The listing builds one solid part. Answer for the finished solid, in the listing's coordinates (mm). Face numbers are marked on the shaded views. A direction names the side the tool comes from. Coordinates: 2 decimals unless noted, no trailing zeros. Write each loop counter-clockwise with the first axis right and the second up, starting at its lowest first coordinate (ties: lowest second). Pieces come first, ordered by that corner, then holes.
from build123d import *

# Parameters (mm, degrees)
BASE_FLANGE1_DEPTH                                  = 50
M12_CLEARANCE_HOLE1_D                               = 12.1
M6_CLEARANCE_HOLE1_D                                = 6.6
BREAK_CORNER1_START                                 = -3
BREAK_CORNER1_DEPTH                                 = 3
BREAK_CORNER1_2_DEPTH                               = 3
EDGE_FLANGE2_DEPTH                                  = 47
CSK_FOR_M8_COUNTERSUNK_FLAT_HEAD_SCREW1_D           = 9
CSK_FOR_M8_COUNTERSUNK_FLAT_HEAD_SCREW1_CSINK_D     = 17.3
CSK_FOR_M8_COUNTERSUNK_FLAT_HEAD_SCREW1_CSINK_ANGLE = 90
CSK_FOR_M6_COUNTERSUNK_FLAT_HEAD_SCREW1_D           = 6.6
CSK_FOR_M6_COUNTERSUNK_FLAT_HEAD_SCREW1_CSINK_D     = 12.6
CSK_FOR_M6_COUNTERSUNK_FLAT_HEAD_SCREW1_CSINK_ANGLE = 90


# Read off the part's stored shape, not the designer's step: Break-Corner1
# Sheet-metal steps are written as plain solids
with BuildPart() as part:
    # Sketch1 → Base-Flange1 (new body)
    with BuildSketch(Plane.XY):
        with BuildLine():
            Line((0, 55), (0, 3))
            ThreePointArc((0, 3), (-0.878679656, 0.878679656), (-3, 0))
            Line((-3, 0), (-30, 0))
            Line((-30, 0), (-30, -3))
            Line((-30, -3), (-3, -3))
            ThreePointArc((-3, -3), (1.242640687, -1.242640687), (3, 3))
            Line((3, 3), (3, 55))
            Line((3, 55), (0, 55))
        make_face()
    extrude(amount=BASE_FLANGE1_DEPTH)

    # M12 Clearance Hole1 (through all)
    with Locations(Plane.ZY):
        with Locations((25, 40)):
            Hole(M12_CLEARANCE_HOLE1_D / 2)

    # M6 Clearance Hole1 (through all)
    with Locations(Plane(origin=(0, 0, 0), x_dir=(1, 0, 0), z_dir=(0, 1, 0))):
        with Locations((-16.5, -40), (-16.5, -10)):
            Hole(M6_CLEARANCE_HOLE1_D / 2)

    # Break-Corner1 outline → Break-Corner1 (cut)
    with BuildSketch(Plane(origin=(0, 0, 0), x_dir=(1, 0, 0), z_dir=(0, 1, 0)).offset(BREAK_CORNER1_START)):
        with BuildLine():
            Line((-30, -50), (-25, -50))
            ThreePointArc((-25, -50), (-28.535533906, -48.535533906), (-30, -45))
            Line((-30, -45), (-30, -50))
        make_face()
        with BuildLine():
            Line((-30, 0), (-30, -5))
            ThreePointArc((-30, -5), (-28.535533906, -1.464466094), (-25, 0))
            Line((-25, 0), (-30, 0))
        make_face()
    extrude(amount=BREAK_CORNER1_DEPTH, mode=Mode.SUBTRACT)

    # Break-Corner1 2 outline → Break-Corner1 2 (cut)
    with BuildSketch(Plane.YZ):
        with BuildLine():
            Line((55, 0), (55, 5))
            ThreePointArc((55, 5), (53.535533906, 1.464466094), (50, 0))
            Line((50, 0), (55, 0))
        make_face()
        with BuildLine():
            ThreePointArc((50, 50), (53.535533906, 48.535533906), (55, 45))
            Line((55, 45), (55, 50))
            Line((55, 50), (50, 50))
        make_face()
    extrude(amount=BREAK_CORNER1_2_DEPTH, mode=Mode.SUBTRACT)

    # Edge-Flange2 section (across the edge) → Edge-Flange2 (add)
    with BuildSketch(Plane(origin=(0, 3, 51.242640687), x_dir=(-0.7071067811865512, 0, -0.7071067811865438), z_dir=(0, 1, 0))):
        with BuildLine():
            Line((-3, 1.242640687), (-3, 42.757359313))
            Line((-3, 42.757359313), (0, 42.757359313))
            Line((0, 42.757359313), (0, 1.242640687))
            ThreePointArc((0, 1.242640687), (0.228361402, 0.09459039), (0.878679656, -0.878679656))
            Line((0.878679656, -0.878679656), (-1.242640687, -3))
            ThreePointArc((-1.242640687, -3), (-2.543277195, -1.053459907), (-3, 1.242640687))
        make_face()
    extrude(amount=EDGE_FLANGE2_DEPTH)

    # CSK for M8 Countersunk Flat Head Screw1 (through all)
    with Locations(Plane(origin=(25.621320344, 0, 25.621320344), x_dir=(-0.7071067811865437, 0, 0.7071067811865513), z_dir=(-0.7071067811865513, 0, -0.7071067811865437))):
        with Locations((68.299943249, 21.537354557)):
            CounterSinkHole(CSK_FOR_M8_COUNTERSUNK_FLAT_HEAD_SCREW1_D / 2, CSK_FOR_M8_COUNTERSUNK_FLAT_HEAD_SCREW1_CSINK_D / 2, counter_sink_angle=CSK_FOR_M8_COUNTERSUNK_FLAT_HEAD_SCREW1_CSINK_ANGLE)

    # CSK for M6 Countersunk Flat Head Screw1 (through all)
    with Locations(Plane(origin=(3, 0, 0), x_dir=(0, 0, -1), z_dir=(1, 0, 0))):
        with Locations((-14.330047328, 16.438814783)):
            CounterSinkHole(CSK_FOR_M6_COUNTERSUNK_FLAT_HEAD_SCREW1_D / 2, CSK_FOR_M6_COUNTERSUNK_FLAT_HEAD_SCREW1_CSINK_D / 2, counter_sink_angle=CSK_FOR_M6_COUNTERSUNK_FLAT_HEAD_SCREW1_CSINK_ANGLE)


solid = part.part
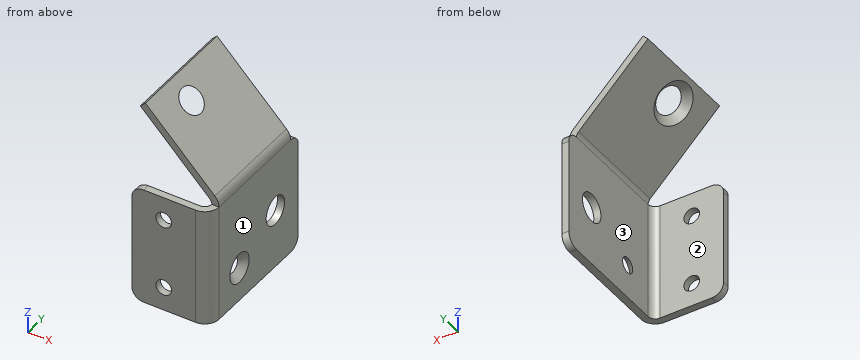
Q1. The part is cut by section D-D, the plane z = 56.5. Write down the section's boundary in (x, y), then the cut area to 3 significant figures.
Answers below:
outline: (-5.26, 3) - (-1.01, 3) - (-1.01, 50) - (-5.26, 50) - close
area: 199 mm2
Q2. The part is cut by section A-A, the plane z = 40. Write down the section's boundary in (x, y), then the cut area to 3 significant figures.
Answers below:
outline: (-30, -3) - (-19.8, -3) - (-19.8, 0) - (-30, 0) - close; (-13.2, -3) - (-3, -3) arc R6 ccw to (3, 3) - (3, 55) - (0, 55) - (0, 3) arc R3 cw to (-3, 0) - (-13.2, 0) - close
area: 238 mm2
Q3. Which of the six approach directions +Z, -Z, +X, -X, +Y, -Y give full straight-line access (tool end or side, diameter ignored) to the marked faces 1, 2 and 3?
Answers below:
face 1: +Z, -Z, +X, +Y, -Y
face 2: +Z, -Z, -X, +Y
face 3: -Z, -X, +Y
Q4. The part is cut by section B-B, the plane y = 40. Write down the section's boundary in (x, z), then the cut area to 3 significant figures.
Answers below:
outline: (-30.23, 81.48) - (-0.88, 52.12) arc R3 cw to (0, 50) - (0, 31.05) - (3, 31.05) - (3, 50) arc R6 ccw to (1.24, 54.24) - (-28.11, 83.6) - close; (0, 0) - (3, 0) - (3, 18.95) - (0, 18.95) - close
area: 249 mm2
Q5. Find the intervals of material crossed by probe 1 along Z at (x, y) = (-16.5, -2.35); probe 2 along X at (y, z) = (22, 8.5); probe 3 along X at (y, z) = (-1, 40), in increasing order.
Answers below:
probe 1: z = 0 to 6.7, 13.3 to 36.7, 43.3 to 50
probe 2: x = 0 to 3
probe 3: x = -30 to -19.8, -13.2 to 1.47
Q6. The part is cut by section C-C, the plane x = -9. Write down the section's boundary in (y, z), then the cut area to 3 significant figures.
Answers below:
outline: (-3, 0) - (0, 0) - (0, 50) - (-3, 50) - close; (3, 60.24) - (50, 60.24) - (50, 64.49) - (3, 64.49) - close
area: 349 mm2
Q7. Given pin 1 (1.5 mm diameter, centred on y = 33, z = 43.5, fed in from -X); pin 2 (8 mm diameter, centred on y = 16, z = 73.5, fed in from +X); pin 3 (12 mm diameter, centred on y = 5, z = 28, fed in from -X), each flat-ended and moving along its own axis, determine where each tip first touches the part or whether it passes through.
Answers below:
pin 1: stops at x = 0
pin 2: stops at x = -14.01
pin 3: stops at x = -30
